```python
from build123d import *

# Parameters (mm, degrees)
F1_DEPTH       = 15.24
F4_D           = 12.7
F4_DEPTH       = 1.271
F4_ON_F2_D     = 12.7
F4_ON_F2_DEPTH = 1.271
F5_W           = 7.62
F5_H           = 25.4
F6_DEPTH       = 25.4


# Not quite as in the source:
# - a feature names something its author has since deleted; it is built from what else it names


with BuildPart() as f1:
    # F0 (on Front) → F1 (new body)
    with BuildSketch(Plane.XZ):
        Polygon((-14.4720045709, -37.1843738795), (13.4679954291, -37.1843738795), (13.4679954291, 27.5043461205), (-14.4720045709, 27.5043461205), (-14.4720045709, 26.2343461205), (12.1979954291, 26.2343461205), (12.1979954291, -35.9143738795), (-14.4720045709, -35.9143738795), align=None)
    extrude(amount=F1_DEPTH)

    # F4 (through all, one way)
    with BuildSketch(Plane.XY.offset(-35.9143738795)):
        with Locations((-1.1370045709, -7.62)):
            Circle(F4_D / 2)
    extrude(amount=-F4_DEPTH, mode=Mode.SUBTRACT)

    # F4 on F2 (through all, one way)
    with BuildSketch(Plane(origin=(0, 0, 26.2343461205), x_dir=(1, 0, 0), z_dir=(0, 0, -1))):
        with Locations((-1.1370045709, 7.62)):
            Circle(F4_ON_F2_D / 2)
    extrude(amount=-F4_ON_F2_DEPTH, mode=Mode.SUBTRACT)

    # F5 (on face) → F6 (cut)
    with BuildSketch(Plane(origin=(12.1979954291, 0, 0), x_dir=(0, -1, 0), z_dir=(-1, 0, 0))):
        with Locations((7.62, -17.5400138795)):
            Rectangle(F5_W, F5_H)
        with Locations((7.62, 7.8599861205)):
            Rectangle(F5_W, F5_H)
    extrude(amount=-F6_DEPTH, mode=Mode.SUBTRACT)


solid = f1.part
```
The model under review builds one solid part; all positions refer to its coordinate system, in mm. A direction names the side the tool comes from. Give positions to 0.01 mm unless a question says otherwise; leave off trailing zeros. Write each loop counter-clockwise with the first axis right and the second up, starting at its lowest first coordinate (ties: lowest second). Pieces come first, ordered by that corner, then holes. Notation, with made-up numbers: M 38,52 L 66,52 A33 ccw 66,88 Z; hole C 9,-38.5 d9. An arc over 180 degrees is marked long. Answer in a Markdown table with one row per item.
Item 1: For line 1 along Z through (x, y) = (-6.5, -11.5); line 2 along X through (y, z) = (-7.62, 26.7); line 3 along X through (y, z) = (-13.75, 6), list the stretches that pass through material, from the lowest coordinate up.
Check sheet entries:
| item | result |
|---|---|
| line 1 | -37.18 to -35.91, 26.23 to 27.5 |
| line 2 | -14.47 to -7.49, 5.21 to 13.47 |
| line 3 | 12.2 to 13.47 |
Item 2: Draft analysis for pull direction Z (two halves, no side actions). For faces 4 (the face through (6, -8, -37.184)), 5 (the face through (13, -15.24, 10)), 6 (the face through (3, -2, 27.504)), 7 (the face through (13, -3.81, -4)), state which applies: +Z half, -Z half, draft (parallel to the pull), parting line (faces both ways), or undercut.
Check sheet entries:
| item | result |
|---|---|
| face 4 | -Z half |
| face 5 | draft |
| face 6 | +Z half |
| face 7 | undercut |
Item 3: Add section D-D on x = -2.5. Give the boundary of the cut face in (y, z), plus the area to 3 significant figures.
Check sheet entries:
| item | result |
|---|---|
| outline | M -15.24,-37.18 L -13.82,-37.18 L -13.82,-35.91 L -15.24,-35.91 Z; M -15.24,26.23 L -13.82,26.23 L -13.82,27.5 L -15.24,27.5 Z; M -1.42,-37.18 L 0,-37.18 L 0,-35.91 L -1.42,-35.91 Z; M -1.42,26.23 L 0,26.23 L 0,27.5 L -1.42,27.5 Z |
| area | 7.20 mm2 |
Item 4: For P1, Ø7.5, axis at y = -7.5, z = -5.5, coming from the -X side; P2, Ø0.6, axis at x = 13, z = 3.5, coming from the +Y side, all flat-tipped, find the tip position at first contact; note any pin that passes through.
Check sheet entries:
| item | result |
|---|---|
| P1 | x = 12.2 |
| P2 | y = 0 |
Item 5: Add section B-B on z = -24. Give the boundary of the cut face in (x, y).
Check sheet entries:
| item | result |
|---|---|
| outline | M 12.2,-15.24 L 13.47,-15.24 L 13.47,-11.43 L 12.2,-11.43 Z; M 12.2,-3.81 L 13.47,-3.81 L 13.47,0 L 12.2,0 Z |
Item 6: Add section C-C on y = -7.62. Give the boundary of the cut face in (x, z).
Check sheet entries:
| item | result |
|---|---|
| outline | M -14.47,-37.18 L -7.49,-37.18 L -7.49,-35.91 L -14.47,-35.91 Z; M -14.47,26.23 L -7.49,26.23 L -7.49,27.5 L -14.47,27.5 Z; M 5.21,-37.18 L 13.47,-37.18 L 13.47,-30.24 L 12.2,-30.24 L 12.2,-35.91 L 5.21,-35.91 Z; M 5.21,26.23 L 12.2,26.23 L 12.2,20.56 L 13.47,20.56 L 13.47,27.5 L 5.21,27.5 Z |
Item 7: Tool access review of faces 1 (the face through (5, -4, -35.914)), 2 (the face through (13, -11.43, -5)), 3 (the face through (-14.472, -8, -37)): name each direction out of +Z, -Z, +X, -X, +Y, -Y from which nothing blocks a thin tool from reaching the whole face with its end or side.
Check sheet entries:
| item | result |
|---|---|
| face 1 | -X, +Y, -Y |
| face 2 | +X, -X |
| face 3 | +Z, -Z, -X, +Y, -Y |
Item 8: Add section A-A on x = -11.75. Give the boundary of the cut face in (y, z).
Check sheet entries:
| item | result |
|---|---|
| outline | M -15.24,-37.18 L 0,-37.18 L 0,-35.91 L -15.24,-35.91 Z; M -15.24,26.23 L 0,26.23 L 0,27.5 L -15.24,27.5 Z |
